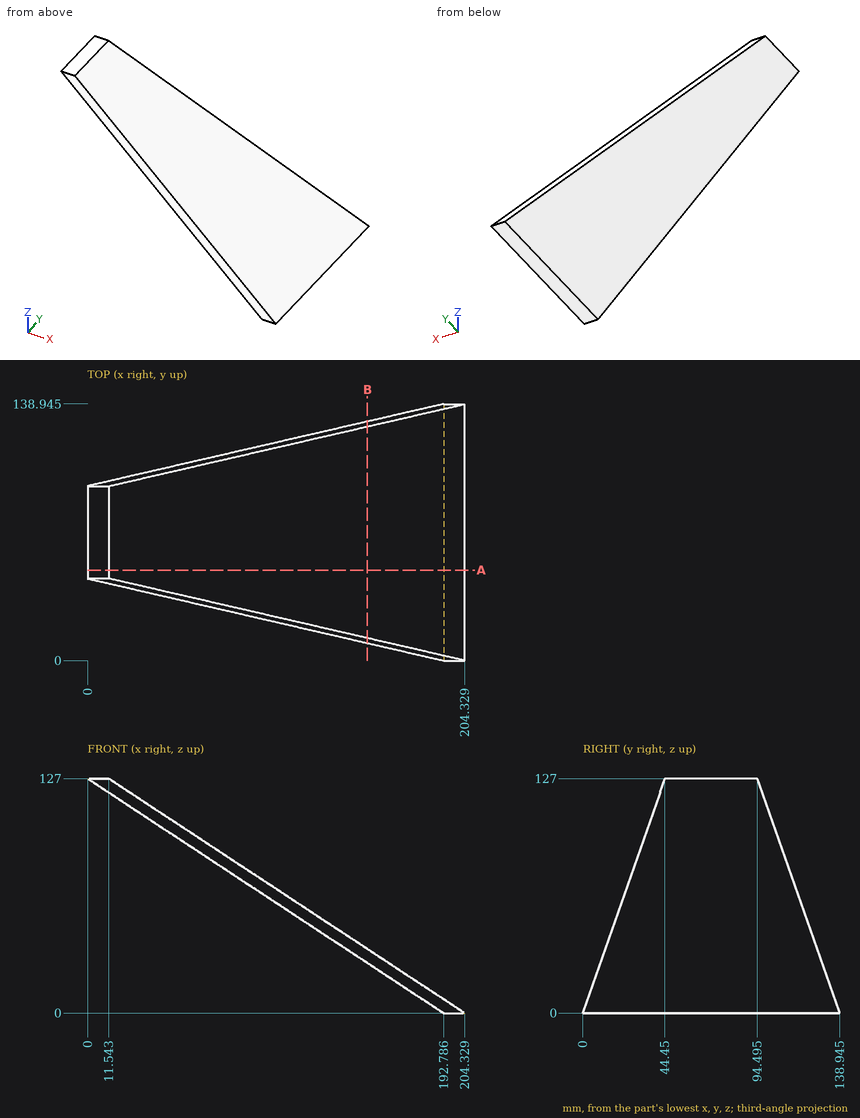
Study the drawing (mm; zero at the part's minimum x, y, z) and answer. Round coordinates to 2 decimals unless told otherwise and drop trailing zeros. Write each loop counter-clockwise with the first axis right and the second up, starting at its lowest first coordinate (ties: lowest second). Pieces come first, ordered by that corner, then holes. Notation, with made-up numbers: (-40, 0.5) - (9, 0.5) arc R35 cw to (9, 39.5) - close; hole circle Ø8 at (-2, -19). An arc over 180 degrees is marked (long way). Use a Markdown table: item, result. Add a question column.
1. Flat-ended cylindrical pins translate along their axes: P1, Ø12, axis at x = 43.5, y = 35.5, coming from the -Z side; P2, Ø1, axis at y = 86, z = 25.5, coming from the -X side; P3, Ø4, axis at y = 57.5, z = 28, coming from the -X side (1 decimal). Find the tip coordinate at first contact, or state that the pin passes through.
2. Consider line 1 (X direction, y = 33.5, z = 35.5) (1 decimal); line 2 (Y direction, x = 20.5, z = 120) (1 decimal); line 3 (Z direction, x = 146, y = 70.5) (1 decimal). Determine where each line is inside the solid, lowest interval first.
3. The part is cut by section A-A (y = 49). Write down the section's boundary in (x, z).
4. The part is cut by section B-B (x = 151.5). Write down the section's boundary in (y, z) (1 decimal).
Reported:
| question | item | result |
|---|---|---|
| 1 | P1 | z = 94.39 |
| 1 | P2 | x = 153.32 |
| 1 | P3 | x = 147.2 |
| 2 | line 1 | 138.9 to 150.4 |
| 2 | line 2 | 42 to 96.9 |
| 2 | line 3 | 30.8 to 38.4 |
| 3 | outline | (0, 127) - (192.79, 0) - (204.33, 0) - (11.54, 127) - close |
| 4 | outline | (9.5, 27.2) - (129.4, 27.2) - (126.8, 34.8) - (12.2, 34.8) - close |
